Input: part model. Units: mm. Frame: model coordinates. Face numbers are marked on the shaded views. A direction names the side the tool comes from. Give positions to 0.01 mm unless a question says otherwise; leave off trailing zeros. Loops run counter-clockwise (first coordinate to the right, second up) from the corner with the lowest first, then second, coordinate; pieces in that order, holes last. Notation, with made-up numbers: (6.25, 6) -> (13.25, 6) arc R21 cw to (13.25, 34) -> close; hole circle Ø7 at (21.5, 50). An arc over 180 degrees is marked (long way). One line per question, with ' | ' between items.
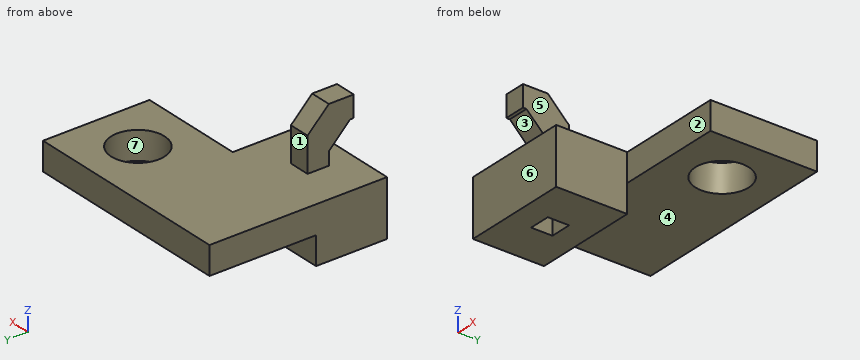
from build123d import *

# Parameters (mm, degrees)
F0_R     = 1.905
F0_W     = 7.62
F0_H     = 5.08
F0_W_2   = 1.524
F0_H_2   = 1.524
F1_DEPTH = 2
F2_DEPTH = 2
F3_DEPTH = 5.9944
F4_W     = 1.524
F4_H     = 1.524
F5_DEPTH = 2.4638
F6_SIZE  = 1.524


# Not quite as in the source:
# - a feature names something its author has since deleted; it is built from what else it names


with BuildPart() as f1:
    # F0 (on Top) → F1 (new body)
    with BuildSketch(Plane.XY):
        Polygon((-32.4838893509, -2.5229738411), (-32.4838893509, 5.0970261589), (-47.7238893509, 5.0970261589), (-47.7238893509, -2.5229738411), (-40.1038893509, -2.5229738411), align=None)
        with Locations((-36.2938893509, 1.2870261589)):
            Circle(F0_R, mode=Mode.SUBTRACT)
        with Locations((-43.9138893509, -5.0629738411)):
            Rectangle(F0_W, F0_H)
        with Locations((-43.9138893509, -5.0629738411)):
            Rectangle(F0_W_2, F0_H_2, mode=Mode.SUBTRACT)
    extrude(amount=F1_DEPTH)

    # F0 (on Top) → F2 (join)
    with BuildSketch(Plane.XY):
        with Locations((-43.9138893509, -5.0629738411)):
            Rectangle(F0_W, F0_H)
        with Locations((-43.9138893509, -5.0629738411)):
            Rectangle(F0_W_2, F0_H_2, mode=Mode.SUBTRACT)
    extrude(amount=-F2_DEPTH)

    # F0 (on Top) → F3 (join)
    with BuildSketch(Plane.XY):
        with Locations((-43.9138893509, -5.0629738411)):
            Rectangle(F0_W_2, F0_H_2)
    extrude(amount=F3_DEPTH)

    # F4 (on face) → F5 (join)
    with BuildSketch(Plane.XZ.offset(7.6029738411)):
        with Locations((-43.9138893509, 5.2324)):
            Rectangle(F4_W, F4_H)
    extrude(amount=-F5_DEPTH)

    # F6
    f6_edges = [f1.edges().sort_by_distance(p)[0] for p in [
        (-43.913889, -5.824974, 4.4704),
        (-43.913889, -4.300974, 5.9944),
    ]]
    chamfer(f6_edges, length=F6_SIZE)


solid = f1.part
1. Section query D-D (x = -40.5). Output: boundary loops of the cut face in (y, z), then the cut area to 3 significant figures.
Determined:
outline: (-7.6, -2) -> (-2.52, -2) -> (-2.52, 0) -> (5.1, 0) -> (5.1, 2) -> (-7.6, 2) -> close | area: 35.6 mm2
2. Section query B-B (y = 2.75). Output: boundary loops of the cut face in (x, z), then the cut area to 3 significant figures.
Determined:
outline: (-47.72, 0) -> (-37.51, 0) -> (-37.51, 2) -> (-47.72, 2) -> close; (-35.07, 0) -> (-32.48, 0) -> (-32.48, 2) -> (-35.07, 2) -> close | area: 25.6 mm2
3. Reachability of the marked faces 1, 2, 3 and 4 from +Z, -Z, +X, -X, +Y, -Y: full face, straight path, thin tool, end or side. Return the list, or none.
Determined:
face 1: +Z, +X, -X, +Y | face 2: +Z, -Z, +X, -Y | face 3: +X, -X, -Y | face 4: -Z, +X, -X, +Y
4. Pin query (flat end, axial travel): P1, Ø1.7, axis at y = -6.5, z = 3, coming from the +X side; P2, Ø1.2, axis at y = -4.5, z = 1, coming from the +X side; P3, Ø2, axis at x = -45.5, z = -1.5, coming from the +Y side. Return the tip coordinate at first contact, or that it passes through.
Determined:
P1: stops at x = -43.15 | P2: stops at x = -40.1 | P3: stops at y = -2.52
5. Section query A-A (z = -1). Output: boundary loops of the cut face in (x, y), then the cut area to 3 significant figures.
Determined:
outline: (-47.72, -7.6) -> (-40.1, -7.6) -> (-40.1, -2.52) -> (-47.72, -2.52) -> close; hole (-44.68, -5.82) -> (-43.15, -5.82) -> (-43.15, -4.3) -> (-44.68, -4.3) -> close | area: 36.4 mm2
6. Pull-direction query (X, two-part tool) for the marked faces 5, 6 and 7; classes: pulls with the +X half, pulls with the -X half, needs draft (parallel to the pull), parting line crosses it, or undercut.
Determined:
face 5: pulls with the +X half | face 6: needs draft | face 7: undercut
7. Section query C-C (x = -35.75). Output: boundary loops of the cut face in (y, z), then the cut area to 3 significant figures.
Determined:
outline: (-2.52, 0) -> (-0.54, 0) -> (-0.54, 2) -> (-2.52, 2) -> close; (3.11, 0) -> (5.1, 0) -> (5.1, 2) -> (3.11, 2) -> close | area: 7.94 mm2
8. Ray query, line 1 along Y through (x, z) = (-43.25, -0.75); line 2 along Y through (x, z) = (-39, 0.25); line 3 along Z through (x, y) = (-41.75, -0.5). Return the intervals inside material, ascending. Write a range as from..to.
Determined:
line 1: y = -7.6..-5.82, -4.3..-2.52 | line 2: y = -2.52..5.1 | line 3: z = 0..2
